from build123d import *

# Parameters (mm, degrees)
PAD_DEPTH       = 12
POCKET_DEPTH    = 4
SKETCH002_R     = 5.25
PAD001_DEPTH    = 20
SKETCH003_R     = 1.4
POCKET001_DEPTH = 28.001


with BuildPart() as part:
    # Sketch001 → Pad (new body)
    with BuildSketch(Plane.XY):
        with BuildLine():
            ThreePointArc((14, 0), (0, 14), (-14, 0))
            Line((-14, 0), (-14, -42))
            ThreePointArc((-14, -42), (0, -56), (14, -42))
            Line((14, -42), (14, 0))
        make_face()
    extrude(amount=PAD_DEPTH)

    # Sketch (on Face6 of Pad) → Pocket (cut)
    with BuildSketch(Plane.XY.offset(12)):
        with BuildLine():
            ThreePointArc((6, -4.5), (0, 7.5), (-6, -4.5))
            ThreePointArc((-3.84916, -7.806116), (-4.666992, -5.985481), (-6, -4.5))
            Line((-3.84916, -7.806116), (-3.84916, -23.506116))
            ThreePointArc((-3.84916, -23.506116), (0.003896, -27.350001), (3.85084, -23.5))
            Line((3.85084, -7.8), (3.85084, -23.5))
            ThreePointArc((6, -4.5), (4.668722, -5.982823), (3.85084, -7.8))
        make_face()
    extrude(amount=-POCKET_DEPTH, mode=Mode.SUBTRACT)

    # Sketch002 (on Face4 of Pocket) → Pad001 (join)
    with BuildSketch(Plane(origin=(0, 0, 0), x_dir=(1, 0, 0), z_dir=(0, 0, -1))):
        with Locations((0, 42)):
            Circle(SKETCH002_R)
    extrude(amount=PAD001_DEPTH)

    # Sketch003 (on Face15 of Pad001) → Pocket001 (cut, through all)
    with BuildSketch(Plane.XY.offset(8)):
        Circle(SKETCH003_R)
        with Locations((0.000838, -23.5)):
            Circle(SKETCH003_R)
    extrude(amount=-POCKET001_DEPTH, mode=Mode.SUBTRACT)


solid = part.part
The listing builds one solid part. Answer for the finished solid, in the listing's coordinates (mm). A direction names the side the tool comes from. Coordinates: 2 decimals unless noted, no trailing zeros. Write each loop counter-clockwise with the first axis right and the second up, starting at its lowest first coordinate (ties: lowest second). Pieces come first, ordered by that corner, then holes. Notation, with made-up numbers: M -19.5,34 L 21.5,34 A38 cw 21.5,73 Z; hole C 5.25,2.5 d4. An arc over 180 degrees is marked long. Put each result on its own line as item: value. Start each with the question number.
1. A cutting plane is placed at C-C on z = -16. Write down the section's boundary in (x, y), then the cut area to 3 significant figures.
2. A cutting plane is placed at D-D on y = -35. Write down the section's boundary in (x, z).
3. Flat-ended cylindrical pins translate along their axes: P1, Ø8, axis at x = -5, z = -7.5, coming from the -Y side; P2, Ø1.5, axis at x = 0, y = -11, coming from the +Z side; P3, Ø6, axis at x = -3.5, z = 6.5, coming from the +Y side. Find the tip coordinate at first contact, or state that the pin passes through.
4. Which of the six approach directions +Z, -Z, +X, -X, +Y, -Y give full straight-line access (tool end or side, diameter ignored) to faces 1 (the cylindrical face through (0, -56, 6)), 2 (the cylindrical face through (-0.683, -47.205, -9.86)), 3 (the cylindrical face through (-4.65, -6.01, 10.03))?
5. For a pull along X with two mould halves and no side action, classify faces 4 (the flat face through (0, -28, 12)), 5 (the cylindrical face through (0.232, 7.496, 10.028)), 6 (the cylindrical face through (4.684, -5.959, 10.028)), 7 (the cylindrical face through (0, 14, 6)) as pulls with the +X half, pulls with the -X half, needs draft (parallel to the pull), parting line crosses it, or undercut.
6. A cutting plane is placed at B-B on y = -20. Write down the section's boundary in (x, z).
7. A cutting plane is placed at A-A on x = 0. Write down the section's boundary in (y, z).
8. Consider line 1 (Y direction, x = 0, z = 2); line 2 (X direction, y = 0, z = 11); line 3 (Z direction, x = -8, y = -30.5). Determine where each line is inside the solid, lowest interval first. Write a range as from..to.
Resolved:
1. outline: C 0,-42 d10.5
1. area: 86.6 mm2
2. outline: M -14,0 L 14,0 L 14,12 L -14,12 Z
3. P1: stops at y = -47.15
3. P2: stops at z = 8
3. P3: stops at y = 13.99
4. face 1: +Z, -Z, -Y
4. face 2: -Z
4. face 3: +Z
5. face 4: needs draft
5. face 5: undercut
5. face 6: undercut
5. face 7: parting line crosses it
6. outline: M -14,0 L 14,0 L 14,12 L 3.85,12 L 3.85,8 L -3.85,8 L -3.85,12 L -14,12 Z
7. outline: M -56,0 L -47.25,0 L -47.25,-20 L -36.75,-20 L -36.75,0 L -24.9,0 L -24.9,8 L -27.35,8 L -27.35,12 L -56,12 Z; M -22.1,0 L -1.4,0 L -1.4,8 L -22.1,8 Z; M 1.4,0 L 14,0 L 14,12 L 7.5,12 L 7.5,8 L 1.4,8 Z
8. line 1: y = -56..-24.9, -22.1..-1.4, 1.4..14
8. line 2: x = -14..-7.5, 7.5..14
8. line 3: z = 0..12
